Check sheet for the drawn part. Datum: minimum x, y, z corner. Units: mm. A direction names the side the tool comes from. Coordinates: 2 decimals unless noted, no trailing zeros. Loops run counter-clockwise (first coordinate to the right, second up) from the corner with the lowest first, then second, coordinate; pieces in that order, holes last. Notation, with made-up numbers: (-7, 39) - (5, 39) arc R22 ccw to (5, 49) - close; hole circle Ø11 at (70, 51). An arc over 180 degrees is marked (long way). Write item = value, one per line. Start each with the question number.
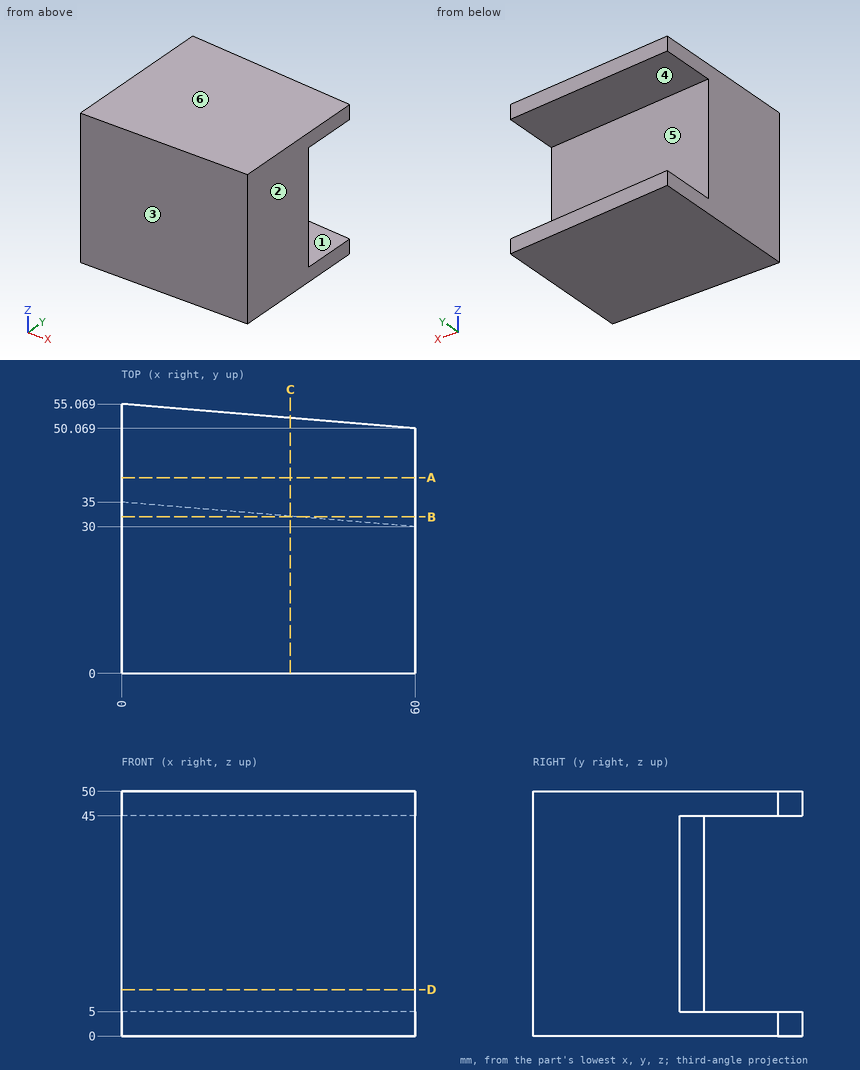
(1) Sectioned sample at C-C on x = 34.5. Enter the section's corners in (y, z) (1 decimal).
(2) Sectioned sample at A-A on y = 40. Enter the section's corners in (x, z), plus the area to 3 significant figures.
(3) Sectioned sample at B-B on y = 32. Enter the section's corners in (x, z), plus the area to 3 significant figures.
(4) Draft check along Z on the marked faces 3, 4, 5 and 6. Enter one of: pulls with the +Z half, pulls with the -Z half, needs draft (parallel to the pull), parting line crosses it, or undercut.
(5) Tool access check on the marked faces 1 and 2. Record the directions out of +Z, -Z, +X, -X, +Y, -Y that give a thin tool (end or side, any length) a straight path to the whole face; none if there is none.
(6) Scan lines: line 1 (Z direction, x = 2.5, y = 38.5); line 2 (Y direction, x = 47, z = 3); line 3 (Y direction, x = 43, z = 30.5). Record each from-to range of solid material in increasing order.
(7) Sectioned sample at D-D on z = 9.5. Enter the section's corners in (x, y).
Working result:
q1.outline = (0, 0) - (52.2, 0) - (52.2, 5) - (32.1, 5) - (32.1, 45) - (52.2, 45) - (52.2, 50) - (0, 50) - close
q2.outline = (0, 0) - (60, 0) - (60, 5) - (0, 5) - close; (0, 45) - (60, 45) - (60, 50) - (0, 50) - close
q2.area = 600 mm2
q3.outline = (0, 0) - (60, 0) - (60, 5) - (36, 5) - (36, 45) - (60, 45) - (60, 50) - (0, 50) - close
q3.area = 2,040 mm2
q4.face_3 = needs draft
q4.face_4 = undercut
q4.face_5 = undercut
q4.face_6 = pulls with the +Z half
q5.face_1 = +X, +Y
q5.face_2 = +Z, -Z, +X, +Y, -Y
q6.line_1 = 0 to 5, 45 to 50
q6.line_2 = 0 to 51.15
q6.line_3 = 0 to 31.42
q7.outline = (0, 0) - (60, 0) - (60, 30) - (0, 35) - close
